```python
from build123d import *

# Parameters (mm, degrees)
F1_DEPTH = 19.6
F2_R     = 6
F3_R     = 3


with BuildPart() as f1:
    # F0 (on Top) → F1 (new body)
    with BuildSketch(Plane.XY):
        Polygon((-28.130636, 0), (-23.030636, 0), (-23.030636, 10), (-12.730636, 10), (-12.730636, 2.5), (-14.530636, 2.5), (-12.730636, 0), (-7.330636, 0), (-7.330636, 7), (6.169364, 5.4), (6.169364, 0), (10.669364, 0), (10.669364, 10.066667), (-7.330636, 12.2), (-27.063274, 12.2), align=None)
    extrude(amount=F1_DEPTH)

    # F2
    f2_edges = [f1.edges().sort_by_distance(p)[0] for p in [
        (10.669364, 10.066667, 9.8),
    ]]
    fillet(f2_edges, radius=F2_R)

    # F3
    f3_edges = [f1.edges().sort_by_distance(p)[0] for p in [
        (-27.063274, 12.2, 9.8),
    ]]
    fillet(f3_edges, radius=F3_R)


solid = f1.part
```
Could you check a few things on this model? Use its own coordinates, in mm. A direction names the side the tool comes from. Round coordinates to 2 decimals unless told otherwise and drop trailing zeros. Loops run counter-clockwise (first coordinate to the right, second up) from the corner with the lowest first, then second, coordinate; pieces in that order, holes last. Notation, with made-up numbers: (-35, 34) - (-19, 34) arc R14 ccw to (-19, 38) - close; hole circle Ø4 at (42, 44). An arc over 180 degrees is marked (long way). Answer in a Markdown table with one row per item. Add a question column.
(1) If we section it at A-A (z = 11.5): Please give me the cut outline in (x, y), plus the area to 3 significant figures.
(2) For faces 1 (the face through (-0.889, 11.437, 9.663)), 2 (the face through (-14, 2.5, 10)), 3 (the face through (-23.031, 5, 10)), which set-ups out of +Z, -Z, +X, -X, +Y, -Y let a thin tool reach every point of the face, with its end or its side?
(3) If we section it at C-C (x = -17): Please give me the cut outline in (y, z).
(4) If we mould it in two halves opening along Y, with no side actions, what happens to faces 4 (the face through (-10, 0, 10)), 5 (the face through (-12.731, 6, 10)), 6 (the face through (-9, 8, 0))? For each: pulls with the +Y half, pulls with the -Y half, needs draft (parallel to the pull), parting line crosses it, or undercut.
(5) I'm going to push flat-ended pins straight in: pin 1 (4 mm diameter, centred on y = 7, z = 14, fed in from -X); pin 2 (1.6 mm diameter, centred on y = 1.5, z = 10.5, fed in from -X); pin 3 (1 mm diameter, centred on y = 8, z = 5.5, fed in from +X). Where does each tip first touch, or does it pass through?
(6) I need wall thicknesses on line 1 along X through (y, z) = (1, 11.25); line 2 along X through (y, z) = (2, 18); line 3 along Y through (x, z) = (-18.5, 13.75). Which ranges of each line are inside material? Lowest first, please.
(7) If we section it at B-B (y = 4.25): Please give me the cut outline in (x, z).
(8) If we section it at D-D (y = 11.25): Please give me the cut outline in (x, z) (3 decimals), plus the area to 3 significant figures.
Model answer:
| question | item | result |
|---|---|---|
| 1 | outline | (-28.13, 0) - (-23.03, 0) - (-23.03, 10) - (-12.73, 10) - (-12.73, 2.5) - (-14.53, 2.5) - (-12.73, 0) - (-7.33, 0) - (-7.33, 7) - (6.17, 5.4) - (6.17, 0) - (10.67, 0) - (10.67, 4.74) arc R6 ccw to (5.38, 10.69) - (-7.33, 12.2) - (-24.31, 12.2) arc R3 ccw to (-27.3, 9.46) - close |
| 1 | area | 256 mm² |
| 2 | face 1 | +Z, -Z, +X, +Y |
| 2 | face 2 | +Z, -Z |
| 2 | face 3 | +Z, -Z, -Y |
| 3 | outline | (10, 0) - (12.2, 0) - (12.2, 19.6) - (10, 19.6) - close |
| 4 | face 4 | pulls with the -Y half |
| 4 | face 5 | undercut |
| 4 | face 6 | needs draft |
| 5 | pin 1 | stops at x = -27.69 |
| 5 | pin 2 | stops at x = -28.07 |
| 5 | pin 3 | stops at x = 9.99 |
| 6 | line 1 | x = -28.04 to -23.03, -13.45 to -7.33, 6.17 to 10.67 |
| 6 | line 2 | x = -27.96 to -23.03, -14.17 to -7.33, 6.17 to 10.67 |
| 6 | line 3 | y = 10 to 12.2 |
| 7 | outline | (-27.76, 0) - (-23.03, 0) - (-23.03, 19.6) - (-27.76, 19.6) - close; (-12.73, 0) - (-7.33, 0) - (-7.33, 19.6) - (-12.73, 19.6) - close; (6.17, 0) - (10.67, 0) - (10.67, 19.6) - (6.17, 19.6) - close |
| 8 | outline | (-26.505, 0) - (0.685, 0) - (0.685, 19.6) - (-26.505, 19.6) - close |
| 8 | area | 533 mm² |
